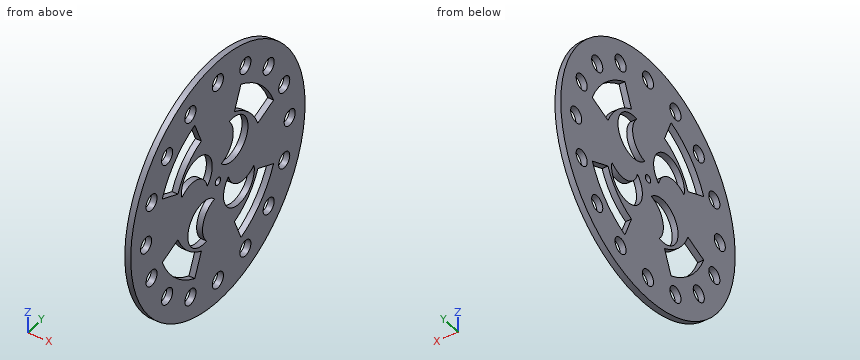
from build123d import *

# Parameters (mm, degrees)
F0_R     = 53.975
F0_R_2   = 3.429
F0_R_3   = 1.651
F1_DEPTH = 2.54


with BuildPart() as f1:
    # F0 (on Right) → F1 (new body)
    with BuildSketch(Plane.YZ):
        Circle(F0_R)
        with Locations((-31.430896, -31.430896)):
            Circle(F0_R_2, mode=Mode.SUBTRACT)
        with Locations((-17.010279, -41.066445)):
            Circle(F0_R_2, mode=Mode.SUBTRACT)
        with Locations((-41.066445, -17.010279)):
            Circle(F0_R_2, mode=Mode.SUBTRACT)
        with BuildLine():
            ThreePointArc((-14.285149, -34.487401), (-26.395514, -26.395514), (-34.487401, -14.285149))
            Line((-34.487401, -14.285149), (-24.757027, -10.254696))
            ThreePointArc((-24.757027, -10.254696), (-18.948208, -18.948208), (-10.254696, -24.757027))
            Line((-10.254696, -24.757027), (-14.285149, -34.487401))
        make_face(mode=Mode.SUBTRACT)
        with BuildLine():
            ThreePointArc((-7.017803, -22.315191), (-18.172542, -10.16), (-2.068468, -6.577309))
            ThreePointArc((-2.068468, -6.577309), (-9.086271, -13.0175), (-7.017803, -22.315191))
        make_face(mode=Mode.SUBTRACT)
        with Locations((0, -44.45)):
            Circle(F0_R_2, mode=Mode.SUBTRACT)
        with Locations((17.010279, -41.066445)):
            Circle(F0_R_2, mode=Mode.SUBTRACT)
        with Locations((31.430896, -31.430896)):
            Circle(F0_R_2, mode=Mode.SUBTRACT)
        with BuildLine():
            ThreePointArc((10.254696, -24.757027), (18.948208, -18.948208), (24.757027, -10.254696))
            Line((24.757027, -10.254696), (34.487401, -14.285149))
            ThreePointArc((34.487401, -14.285149), (26.395514, -26.395514), (14.285149, -34.487401))
            Line((14.285149, -34.487401), (10.254696, -24.757027))
        make_face(mode=Mode.SUBTRACT)
        with BuildLine():
            ThreePointArc((22.315191, -7.017803), (10.16, -18.172542), (6.577309, -2.068468))
            ThreePointArc((6.577309, -2.068468), (13.0175, -9.086271), (22.315191, -7.017803))
        make_face(mode=Mode.SUBTRACT)
        with Locations((41.066445, -17.010279)):
            Circle(F0_R_2, mode=Mode.SUBTRACT)
        with Locations((-44.45, 0)):
            Circle(F0_R_2, mode=Mode.SUBTRACT)
        with Locations((-41.066445, 17.010279)):
            Circle(F0_R_2, mode=Mode.SUBTRACT)
        with BuildLine():
            ThreePointArc((-22.315191, 7.017803), (-10.16, 18.172542), (-6.577309, 2.068468))
            ThreePointArc((-6.577309, 2.068468), (-13.0175, 9.086271), (-22.315191, 7.017803))
        make_face(mode=Mode.SUBTRACT)
        with BuildLine():
            ThreePointArc((-34.487401, 14.285149), (-26.395514, 26.395514), (-14.285149, 34.487401))
            Line((-14.285149, 34.487401), (-10.254696, 24.757027))
            ThreePointArc((-10.254696, 24.757027), (-18.948208, 18.948208), (-24.757027, 10.254696))
            Line((-24.757027, 10.254696), (-34.487401, 14.285149))
        make_face(mode=Mode.SUBTRACT)
        with Locations((-31.430896, 31.430896)):
            Circle(F0_R_2, mode=Mode.SUBTRACT)
        with Locations((-17.010279, 41.066445)):
            Circle(F0_R_2, mode=Mode.SUBTRACT)
        Circle(F0_R_3, mode=Mode.SUBTRACT)
        with BuildLine():
            ThreePointArc((7.017803, 22.315191), (18.172542, 10.16), (2.068468, 6.577309))
            ThreePointArc((2.068468, 6.577309), (9.086271, 13.0175), (7.017803, 22.315191))
        make_face(mode=Mode.SUBTRACT)
        with BuildLine():
            Line((34.487401, 14.285149), (24.757027, 10.254696))
            ThreePointArc((24.757027, 10.254696), (18.948208, 18.948208), (10.254696, 24.757027))
            Line((10.254696, 24.757027), (14.285149, 34.487401))
            ThreePointArc((14.285149, 34.487401), (26.395514, 26.395514), (34.487401, 14.285149))
        make_face(mode=Mode.SUBTRACT)
        with Locations((44.45, 0)):
            Circle(F0_R_2, mode=Mode.SUBTRACT)
        with Locations((41.066445, 17.010279)):
            Circle(F0_R_2, mode=Mode.SUBTRACT)
        with Locations((0, 44.45)):
            Circle(F0_R_2, mode=Mode.SUBTRACT)
        with Locations((17.010279, 41.066445)):
            Circle(F0_R_2, mode=Mode.SUBTRACT)
        with Locations((31.430896, 31.430896)):
            Circle(F0_R_2, mode=Mode.SUBTRACT)
    extrude(amount=F1_DEPTH)


solid = f1.part
Build history of the part. All positions in model axes, mm. Round coordinates to 2 decimals unless told otherwise and drop trailing zeros. Loops run counter-clockwise (first coordinate to the right, second up) from the corner with the lowest first, then second, coordinate; pieces in that order, holes last. Notation, with made-up numbers: (87.25, 41) -> (129.25, 41) arc R18 ccw to (129.25, 65) -> close; hole circle Ø5 at (5, 54.25). An arc over 180 degrees is marked (long way). Answer in a Markdown table with one row per item.
Item 1: Saw through at D-D (x = 2.15). State how many separate pieces and enclosed holes the cut face has, and give its area (3 significant figures).
Answers below:
| item | result |
|---|---|
| separate pieces | 1 |
| enclosed holes | 25 |
| area | 6,800 mm² |
Item 2: Saw through at C-C (y = -16). Write the cut outline in (x, z), and give its area (3 significant figures).
Answers below:
| item | result |
|---|---|
| outline | (0, -51.55) -> (2.54, -51.55) -> (2.54, -44.34) -> (0, -44.34) -> close; (0, -37.79) -> (2.54, -37.79) -> (2.54, -33.73) -> (0, -33.73) -> close; (0, -21.5) -> (2.54, -21.5) -> (2.54, -19.57) -> (0, -19.57) -> close; (0, -6.47) -> (2.54, -6.47) -> (2.54, 9.52) -> (0, 9.52) -> close; (0, 18.13) -> (2.54, 18.13) -> (2.54, 21.5) -> (0, 21.5) -> close; (0, 33.73) -> (2.54, 33.73) -> (2.54, 37.79) -> (0, 37.79) -> close; (0, 44.34) -> (2.54, 44.34) -> (2.54, 51.55) -> (0, 51.55) -> close |
| area | 111 mm² |
Item 3: Pin check, flat tips, straight feed: pin 1 (4 mm diameter, centred on y = 0, z = 0, fed in from -X); pin 2 (1.5 mm diameter, centred on x = 1.5, y = -18.5, fed in from +Z); pin 3 (1 mm diameter, centred on x = 0.5, y = -4, fed in from -Z). Stop position of each tip, or through.
Answers below:
| item | result |
|---|---|
| pin 1 | stops at x = 0 |
| pin 2 | stops at z = 50.97 |
| pin 3 | stops at z = -53.86 |
Item 4: Drill centre lines: L1, parallel to Z at x = 0.95, y = 0 (3 decimals); L2, parallel to Z at x = 1.1, y = -21; L3, parallel to Z at x = 0.75, y = 6. Where is each one in solid material? Low to high. Write a range as [from, to].
Answers below:
| item | result |
|---|---|
| L1 | z = [-53.975, -47.879], [-41.021, -1.651], [1.651, 41.021], [47.879, 53.975] |
| L2 | z = [-49.72, -30.86], [-16.65, 8.03], [14.28, 16.65], [30.86, 49.72] |
| L3 | z = [-53.64, -15.53], [-2.65, 4.01], [8.48, 53.64] |
Item 5: Saw through at A-A (y = 0). Write the cut outline in (x, z) (3 decimals), and give its area (3 significant figures).
Answers below:
| item | result |
|---|---|
| outline | (0, -53.975) -> (2.54, -53.975) -> (2.54, -47.879) -> (0, -47.879) -> close; (0, -41.021) -> (2.54, -41.021) -> (2.54, -1.651) -> (0, -1.651) -> close; (0, 1.651) -> (2.54, 1.651) -> (2.54, 41.021) -> (0, 41.021) -> close; (0, 47.879) -> (2.54, 47.879) -> (2.54, 53.975) -> (0, 53.975) -> close |
| area | 231 mm² |
